```python
from build123d import *

# Parameters (mm, degrees)
SKETCH_1_R          = 28.5
EXTRUDE_1_DEPTH     = 45
SKETCH_2_R          = 17.5
CUT_EXTRUDE_2_DEPTH = 4
SKETCH_2_5_R        = 1.5
CUT_EXTRUDE_3_DEPTH = 5
SKETCH_4_R          = 1.5
CUT_EXTRUDE_4_DEPTH = 4
SKETCH_9_W          = 14
SKETCH_9_H          = 5
CUT_EXTRUDE_6_DEPTH = 3
SKETCH_10_W         = 8
SKETCH_10_H         = 8
CUT_EXTRUDE_7_DEPTH = 3


with BuildPart() as part:
    # 草图1 → 凸台-拉伸1 (new body)
    with BuildSketch(Plane.XY):
        Circle(SKETCH_1_R)
    extrude(amount=EXTRUDE_1_DEPTH)

    # 草图2 → 切除-拉伸2 (cut)
    with BuildSketch(Plane.XY.offset(45)):
        Circle(SKETCH_2_R)
    extrude(amount=-CUT_EXTRUDE_2_DEPTH, mode=Mode.SUBTRACT)

    # 草图2<5> → 切除-拉伸3 (cut)
    with BuildSketch(Plane.XY.offset(45)):
        with Locations((0, 25)):
            Circle(SKETCH_2_5_R)
        with Locations((21.650635095, 12.5)):
            Circle(SKETCH_2_5_R)
        with Locations((21.650635095, -12.5)):
            Circle(SKETCH_2_5_R)
        with Locations((0, -25)):
            Circle(SKETCH_2_5_R)
        with Locations((-21.650635095, -12.5)):
            Circle(SKETCH_2_5_R)
        with Locations((-21.650635095, 12.5)):
            Circle(SKETCH_2_5_R)
    extrude(amount=-CUT_EXTRUDE_3_DEPTH, mode=Mode.SUBTRACT)

    # 草图4 → 切除-拉伸4 (cut)
    with BuildSketch(Plane(origin=(0, 0, 0), x_dir=(-1, 0, 0), z_dir=(0, 0, -1))):
        with Locations((13.435028843, 13.435028843)):
            Circle(SKETCH_4_R)
        with Locations((-13.435028843, 13.435028843)):
            Circle(SKETCH_4_R)
        with Locations((13.435028843, -13.435028843)):
            Circle(SKETCH_4_R)
        with Locations((-13.435028843, -13.435028843)):
            Circle(SKETCH_4_R)
    extrude(amount=-CUT_EXTRUDE_4_DEPTH, mode=Mode.SUBTRACT)

    # 草图9 → 切除-拉伸6 (cut)
    with BuildSketch(Plane(origin=(0, 28.5, 0), x_dir=(1, 0, 0), z_dir=(0, 1, 0))):
        with Locations((0, -3.5)):
            Rectangle(SKETCH_9_W, SKETCH_9_H)
    cut_extrude_6 = extrude(amount=-CUT_EXTRUDE_6_DEPTH, mode=Mode.SUBTRACT)

    # 镜向1: 切除-拉伸6 across plane
    add(cut_extrude_6.mirror(Plane.ZX), mode=Mode.SUBTRACT)

    # 草图10 → 切除-拉伸7 (cut)
    with BuildSketch(Plane(origin=(-28.5, 0, 0), x_dir=(0, 0, -1), z_dir=(1, 0, 0))):
        with Locations((-5, 0)):
            Rectangle(SKETCH_10_W, SKETCH_10_H)
    extrude(amount=CUT_EXTRUDE_7_DEPTH, mode=Mode.SUBTRACT)


solid = part.part
```
Can you work these out from the model? Positions are in its coordinate system, mm. A direction names the side the tool comes from. Coordinates: 2 decimals unless noted, no trailing zeros. Loops run counter-clockwise (first coordinate to the right, second up) from the corner with the lowest first, then second, coordinate; pieces in that order, holes last. Notation, with made-up numbers: (18, -2.75) - (62, -2.75) arc R6 cw to (62, 4.25) - close; hole circle Ø3 at (77.25, 72.5). An arc over 180 degrees is marked (long way). Answer as CSV lines item,"result". Start each with the question number.
1) Which directions (+Z, -Z, +X, -X, +Y, -Y) give clear straight access to the entire face, cutting with the end or side of a thin tool? Please do faces 3 (the flat face through (13, -13, 4)), 4 (the flat face through (0, 27, 6)), 5 (the cylindrical face through (23.08, 12.95, 42.54)).
2) Suppose I cut it at D-D (x = -21). Please give me the cut outline in (y, z).
3) Suppose I cut it at C-C (z = 26). Please give me the cut outline in (x, y).
4) For pin 1 (2 mm diameter, centred on x = -27, z = 3, fed in from +Y); pin 2 (1.5 mm diameter, centred on x = -14, y = -13, fed in from -Z); pin 3 (1.7 mm diameter, centred on y = -26.5, z = 2.5, fed in from -X), each with a flat end and sliding along its axis, tell me the tip position at first contact or that it passes through.
5) Suppose I cut it at A-A (x = 0). Please give me the cut outline in (y, z).
6) Thinking about a two-plate mould opening in X: for faces 1 (the cylindrical face through (12.05, -14.01, 1.97)), 2 (the flat face through (-13, -12, 45)), which applies, pulls with the +X half, pulls with the -X half, needs draft (parallel to the pull), parting line crosses it, or undercut?
7) I need wall thicknesses on line 1 (Y direction, x = 0, z = 42.2); line 2 (Z direction, x = -6, y = 13.5); line 3 (X direction, y = 0, z = 8). Which ranges of each line are inside material? Lowest first, please. Write a range as from..to.
8) Suppose I cut it at B-B (y = 0). Please give me the cut outline in (x, z), plus the area to 3 significant figures.
Check result:
1,face 3,"-Z"
1,face 4,"+Y"
1,face 5,"+Z"
2,outline,"(-19.27, 0) - (19.27, 0) - (19.27, 45) - (13.85, 45) - (13.85, 40) - (11.15, 40) - (11.15, 45) - (-11.15, 45) - (-11.15, 40) - (-13.85, 40) - (-13.85, 45) - (-19.27, 45) - close"
3,outline,"circle Ø57 at (0, 0)"
4,pin 1,"stops at y = 11.67"
4,pin 2,"stops at z = 4"
4,pin 3,"stops at x = -12.42"
5,outline,"(-28.5, 0) - (28.5, 0) - (28.5, 1) - (25.5, 1) - (25.5, 6) - (28.5, 6) - (28.5, 45) - (26.5, 45) - (26.5, 40) - (23.5, 40) - (23.5, 45) - (17.5, 45) - (17.5, 41) - (-17.5, 41) - (-17.5, 45) - (-23.5, 45) - (-23.5, 40) - (-26.5, 40) - (-26.5, 45) - (-28.5, 45) - (-28.5, 6) - (-25.5, 6) - (-25.5, 1) - (-28.5, 1) - close"
6,face 1,"undercut"
6,face 2,"needs draft"
7,line 1,"y = -28.5..-26.5, -23.5..-17.5, 17.5..23.5, 26.5..28.5"
7,line 2,"z = 0..41"
7,line 3,"x = -25.5..28.5"
8,outline,"(-28.5, 0) - (28.5, 0) - (28.5, 45) - (17.5, 45) - (17.5, 41) - (-17.5, 41) - (-17.5, 45) - (-28.5, 45) - (-28.5, 9) - (-25.5, 9) - (-25.5, 1) - (-28.5, 1) - close"
8,area,"2,400 mm²"
